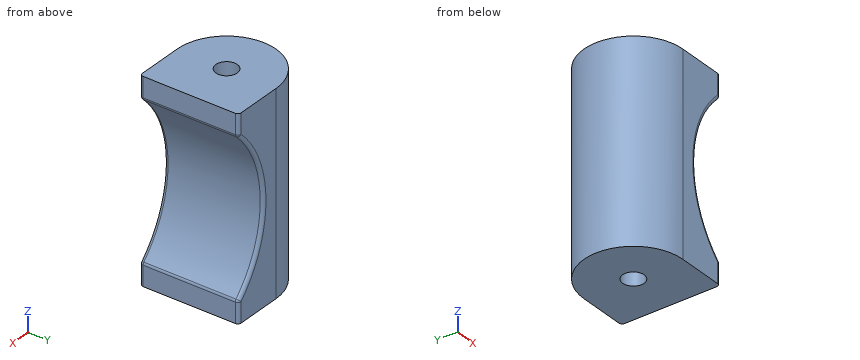
```python
from build123d import *

# Parameters (mm, degrees)
F0_R     = 6.5
F1_DEPTH = 60
F2_R     = 65
F3_DEPTH = 60
F4_R     = 2


with BuildPart() as f1:
    # F0 (on Top) → F1 (new body, symmetric)
    with BuildSketch(Plane.XY):
        with BuildLine():
            Line((30, 30), (0, 30))
            ThreePointArc((0, 30), (21.2132034356, 21.2132034356), (30, 0))
            Line((30, 0), (30, 30))
        make_face()
        with BuildLine():
            ThreePointArc((30, 0), (21.2132034356, 21.2132034356), (0, 30))
            ThreePointArc((0, 30), (-30, 0), (0, -30))
            ThreePointArc((0, -30), (21.2132034356, -21.2132034356), (30, 0))
        make_face()
        Circle(F0_R, mode=Mode.SUBTRACT)
        with BuildLine():
            Line((30, -30), (30, 0))
            ThreePointArc((30, 0), (21.2132034356, -21.2132034356), (0, -30))
            Line((0, -30), (30, -30))
        make_face()
    extrude(amount=F1_DEPTH, both=True)

    # F2 (on Front) → F3 (cut, symmetric)
    with BuildSketch(Plane.XZ):
        with Locations((75, 0)):
            Circle(F2_R)
    extrude(amount=F3_DEPTH, both=True, mode=Mode.SUBTRACT)

    # F4
    f4_edges = [f1.edges().sort_by_distance(p)[0] for p in [
        (10, -30, 0),
        (30, -30, 53.452079),
        (30, 0, -46.904158),
        (30, 0, 46.904158),
        (30, 30, 53.452079),
        (10, 30, 0),
        (30, -30, -53.452079),
        (30, 30, -53.452079),
    ]]
    fillet(f4_edges, radius=F4_R)


solid = f1.part
```
Work out the finished part from the listing and answer in its coordinate system (mm). Coordinates: 2 decimals unless noted, no trailing zeros. Loops run counter-clockwise (first coordinate to the right, second up) from the corner with the lowest first, then second, coordinate; pieces in that order, holes last.
1) Consider probe 1 along X at (y, z) = (1.5, -29); probe 2 along Z at (x, y) = (27, -18.5); probe 3 along Y at (x, z) = (-0.5, -30). Determine where each line is inside the solid, lowest interval first.
Results:
probe 1: x = -29.96 to -6.32, 6.32 to 16.83
probe 2: z = -60 to -43.83, 43.83 to 60
probe 3: y = -30 to -6.48, 6.48 to 30
2) Section D-D (y = -12) is taken. Give the vertices of the cut face in (x, z).
Results:
outline: (-27.5, -60) - (30, -60) - (30, -47.75) arc R2 ccw to (29.4, -46.32) arc R65 cw to (29.4, 46.32) arc R2 ccw to (30, 47.75) - (30, 60) - (-27.5, 60) - close
3) Section A-A (y = 0) is taken. Give the vertices of the cut face in (x, z).
Results:
outline: (-30, -60) - (-6.5, -60) - (-6.5, 60) - (-30, 60) - close; (6.5, -60) - (30, -60) - (30, -47.75) arc R2 ccw to (29.4, -46.32) arc R65 cw to (29.4, 46.32) arc R2 ccw to (30, 47.75) - (30, 60) - (6.5, 60) - close
4) Section C-C (x = -13) is taken. Give the vertices of the cut face in (y, z).
Results:
outline: (-27.04, -60) - (27.04, -60) - (27.04, 60) - (-27.04, 60) - close
5) Flat-ended cylindrical pins translate along their axes: pin 1 (2 mm diameter, centred on x = -14.5, z = -40, fed in from +Y); pin 2 (10 mm diameter, centred on x = -21, z = -14.5, fed in from +Y); pin 3 (10 mm diameter, centred on y = -12.5, z = 21, fed in from +X); pin 4 (10.5 mm diameter, centred on x = 0, y = 0, fed in from -Z). Find the tip coordinate at first contact, or state that the pin passes through.
Results:
pin 1: stops at y = 26.79
pin 2: stops at y = 25.38
pin 3: stops at x = 15.43
pin 4: passes through
6) Section B-B (y = 15.5) is taken. Give the vertices of the cut face in (x, z), plus the area to 3 significant figures.
Results:
outline: (-25.69, -60) - (30, -60) - (30, -47.75) arc R2 ccw to (29.4, -46.32) arc R65 cw to (29.4, 46.32) arc R2 ccw to (30, 47.75) - (30, 60) - (-25.69, 60) - close
area: 5,390 mm2
